Part print with two shaded views. Sizes in mm from the minimum x, y, z corner. A direction names the side the tool comes from. Give positions to 0.01 mm unless a question says otherwise; leave off trailing zeros. Order: outer loops, then holes, each group sorted by start corner. A loop starts at its lowest first (then second) coordinate and runs counter-clockwise, first axis right, second up.
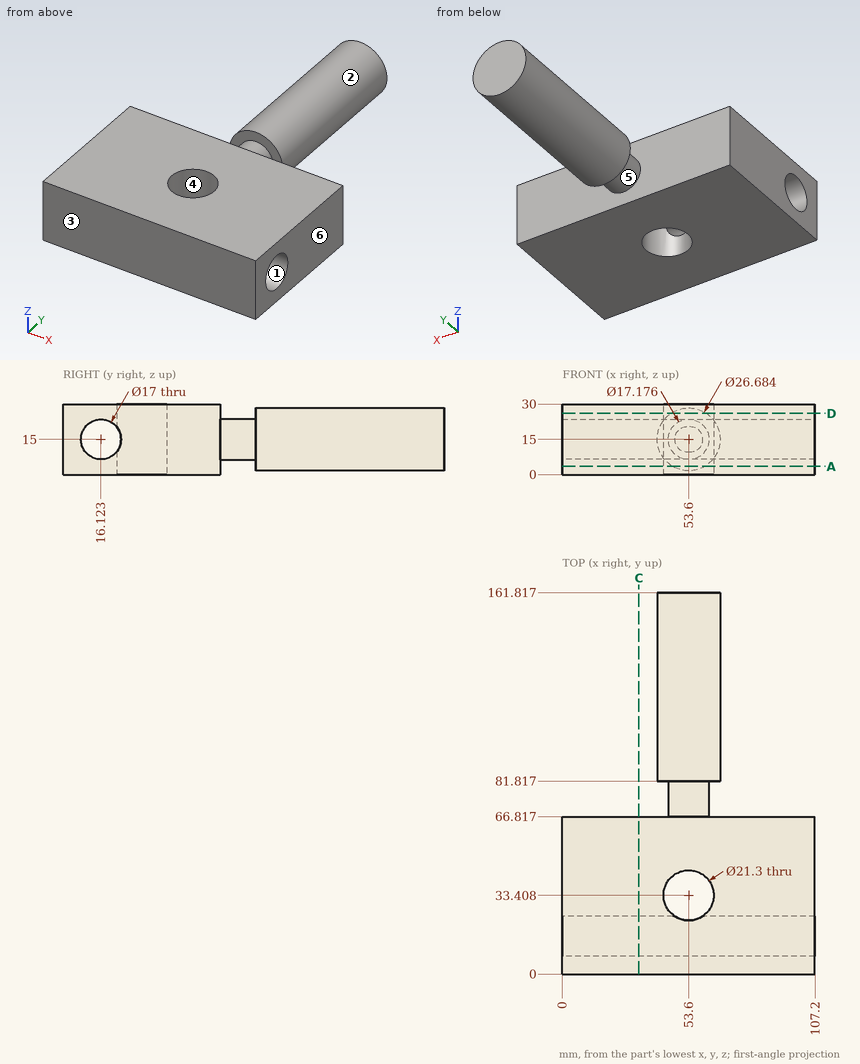
Item 1: Two-plate mould, pull along Y, no slides. Class the marked faces 1, 2, 3 and 4: released by +Y, released by -Y, zero draft, split by the parting line, or undercut.
Item 2: Slice it at C-C (x = 32.5). Give the cut face in (y, z).
Item 3: Wall check: L1, parallel to Y at x = 41.5, z = 14.5; L2, parallel to Y at x = 39, z = 15; L3, parallel to Y at x = 52, z = 5.5. Give the ranges that are in metal, low to high.
Item 4: Drop flat-ended pins along their axis: pin 1 Ø10 at (y, z) = (132, 22) entering from +X; pin 2 Ø8 at (x, y) = (41, 113.5) entering from +Z; pin 3 Ø4 at (x, y) = (55, 133) entering from +Z. Give the stop position or say it passes through.
Item 5: Slice it at D-D (z = 26). Give the cut face in (x, y).
Item 6: Slice it at A-A (z = 3.5). State how many separate pieces and enclosed holes the cut face has, and give its area (3 significant figures).
Item 7: Tool access for the marked faces 5 and 6: list every direction of +Z, -Z, +X, -X, +Y, -Y with a clear straight run to the whole face (end or side of a thin tool).
A:
1. face 1: undercut
1. face 2: zero draft
1. face 3: released by -Y
1. face 4: undercut
2. outline: (0, 0) - (66.82, 0) - (66.82, 30) - (0, 30) - close; hole circle Ø17 at (16.12, 15)
3. L1: y = 0 to 7.64, 24.61 to 66.82, 81.82 to 161.82
3. L2: y = 0 to 7.62, 24.62 to 66.82
3. L3: y = 0 to 22.88, 43.94 to 66.82, 81.82 to 161.82
4. pin 1: stops at x = 66.79
4. pin 2: stops at z = 25.2
4. pin 3: stops at z = 28.34
5. outline: (0, 0) - (107.2, 0) - (107.2, 66.82) - (0, 66.82) - close; (46.05, 81.82) - (61.15, 81.82) - (61.15, 161.82) - (46.05, 161.82) - close; hole circle Ø21.3 at (53.6, 33.41)
6. separate pieces: 2
6. enclosed holes: 1
6. area: 7,890 mm2
7. face 5: none
7. face 6: +Z, -Z, +X, +Y, -Y
